```python
from build123d import *

# Parameters (mm, degrees)
BOSS_EXTRUDE1_DEPTH     = 1
SKETCH2_W               = 20
SKETCH2_H               = 30
BOSS_EXTRUDE2_DEPTH     = 1
MIRROR1_START           = 1
MIRROR1_DEPTH           = 1
MIRROR1_START_2         = 19
MIRROR1_2_DEPTH         = 1
FILLET1_R               = 1
CUT_EXTRUDE1_DEPTH      = 44.502679315
CUT_EXTRUDE1_DEPTH_BACK = 44.502679315
SKETCH3_R               = 2.5
CUT_EXTRUDE2_DEPTH      = 44.502679315
CUT_EXTRUDE2_DEPTH_BACK = 44.502679315
SKETCH4_W               = 27.584874686
SKETCH4_H               = 17.882608418


# Read off the part's stored shape, not the designer's step: Mirror1
with BuildPart() as part:
    # Sketch1 → Boss-Extrude1 (new body)
    with BuildSketch(Plane(origin=(0, 0, 0), x_dir=(0, 0, -1), z_dir=(1, 0, 0))):
        Polygon((0, 24.340975897), (30, 24.340975897), (0, -5.659024103), align=None)
    extrude(amount=BOSS_EXTRUDE1_DEPTH)

    # Sketch2 → Boss-Extrude2 (add)
    with BuildSketch(Plane(origin=(0, 24.340975897, 0), x_dir=(1, 0, 0), z_dir=(0, 1, 0))):
        with Locations((10, 15)):
            Rectangle(SKETCH2_W, SKETCH2_H)
    extrude(amount=-BOSS_EXTRUDE2_DEPTH)

    # Mirror1 outline → Mirror1 (add)
    with BuildSketch(Plane.YZ.offset(MIRROR1_START)):
        Polygon((-5.659024103, 0), (23.340975897, -29), (23.340975897, 0), align=None)
    extrude(amount=MIRROR1_DEPTH)

    # Mirror1 2 outline → Mirror1 2 (add)
    with BuildSketch(Plane.YZ.offset(MIRROR1_START_2)):
        Polygon((-5.659024103, 0), (23.340975897, -29), (23.340975897, 0), align=None)
    extrude(amount=MIRROR1_2_DEPTH)

    # Fillet1
    fillet1_edges = [part.edges().sort_by_distance(p)[0] for p in [
        (20, 24.340975897, -15),
        (19, 23.340975897, -14.5),
        (0, 24.340975897, -15),
        (2, 23.340975897, -14.5),
    ]]
    fillet(fillet1_edges, radius=FILLET1_R - 0.0001)  # a hair under: the kernel refuses the full size

    # Sketch3 → Cut-Extrude1 (cut, two sides: drawn at the far end of the back side and taken through both)
    with BuildSketch(Plane.ZY.offset(-CUT_EXTRUDE1_DEPTH_BACK)):
        with Locations((-5.377949805, 12.578820342)):
            Circle(SKETCH3_R)
    extrude(amount=CUT_EXTRUDE1_DEPTH + CUT_EXTRUDE1_DEPTH_BACK, mode=Mode.SUBTRACT)

    # Sketch4 → Cut-Extrude2 (cut, two sides: drawn at the far end of the back side and taken through both)
    with BuildSketch(Plane.ZY.offset(-CUT_EXTRUDE2_DEPTH_BACK)):
        with Locations((-7.379594799, -1.984577464)):
            Rectangle(SKETCH4_W, SKETCH4_H)
    extrude(amount=CUT_EXTRUDE2_DEPTH + CUT_EXTRUDE2_DEPTH_BACK, mode=Mode.SUBTRACT)


solid = part.part
```
Check sheet for the modelled part. Datum: model origin and axes. Units: mm. A direction names the side the tool comes from. Round coordinates to 2 decimals unless told otherwise and drop trailing zeros. Order: outer loops, then holes, each group sorted by start corner. A loop starts at its lowest first (then second) coordinate and runs counter-clockwise, first axis right, second up. Notation, with made-up numbers: M 8.5,70.5 L 38.5,70.5 A3 cw 38.5,75.5 Z; hole C -10.75,-35 d5. An arc over 180 degrees is marked long. Answer in a Markdown table with one row per item.
(1) Section check C-C on y = 14.5. Record the boundary of the cut face in (x, z).
Findings:
| item | result |
|---|---|
| outline | M 0,-20.16 L 2,-20.16 L 2,-6.98 L 0,-6.98 Z; M 0,-3.78 L 2,-3.78 L 2,0 L 0,0 Z; M 19,-20.16 L 20,-20.16 L 20,-6.98 L 19,-6.98 Z; M 19,-3.78 L 20,-3.78 L 20,0 L 19,0 Z |
(2) Material ranges on line 1 along X through (y, z) = (20.75, -25); line 2 along Y through (x, z) = (17, -3.5); line 3 along Z through (x, y) = (1, 12), recorded low to high. Write a range as from..to.
Findings:
| item | result |
|---|---|
| line 1 | x = 0..2, 19..20 |
| line 2 | y = 23.34..24.34 |
| line 3 | z = -17.66..-7.81, -2.95..0 |
(3) Section check A-A on z = -9. Record the boundary of the cut face in (x, y), plus the area to 3 significant figures.
Findings:
| item | result |
|---|---|
| outline | M 0,6.96 L 2,6.96 L 2,22.34 A1 cw 3,23.34 L 18,23.34 A1 cw 19,22.34 L 19,6.96 L 20,6.96 L 20,23.34 A1 ccw 19,24.34 L 1,24.34 A1 ccw 0,23.34 Z |
| area | 69.2 mm^2 |
(4) Gauge pin test, flat ends, axial feed: pin 1 (4 mm diameter, centred on x = 16, z = -13, fed in from -Y); pin 2 (4.5 mm diameter, centred on y = 12.58, z = -5.38, fed in from +X); pin 3 (4 mm diameter, centred on x = 3, z = -24, fed in from -Y). Record the tip position at first contact, or that the pin passes through.
Findings:
| item | result |
|---|---|
| pin 1 | stops at y = 23.34 |
| pin 2 | passes through |
| pin 3 | stops at y = 16.61 |
(5) Section check B-B on y = 17.5. Record the boundary of the cut face in (x, z), plus the area to 3 significant figures.
Findings:
| item | result |
|---|---|
| outline | M 0,-23.16 L 2,-23.16 L 2,0 L 0,0 Z; M 19,-23.16 L 20,-23.16 L 20,0 L 19,0 Z |
| area | 69.5 mm^2 |
(6) Draft check along X on faces 1 (the flat face through (1, 6.957, -6)), 2 (the cylindrical face through (19.715, 24.04, -15.21)), 3 (the cylindrical face through (18.715, 23.04, -14.297)). Enter one of: +X half, -X half, draft (parallel to the pull), parting line (faces both ways), or undercut.
Findings:
| item | result |
|---|---|
| face 1 | draft |
| face 2 | +X half |
| face 3 | undercut |
(7) Set-up check for faces 4 (the flat face through (19, 16, -11)), 5 (the flat face through (10, 24, -30)): record each of +Z, -Z, +X, -X, +Y, -Y from which the full face is reachable in a straight line by a thin tool's end or side.
Findings:
| item | result |
|---|---|
| face 4 | +Z, -Z, -Y |
| face 5 | -Z, +X, -X, +Y, -Y |
(8) Section check D-D on z = -4. Record the boundary of the cut face in (x, y), plus the area to 3 significant figures.
Findings:
| item | result |
|---|---|
| outline | M 0,6.96 L 2,6.96 L 2,10.49 L 0,10.49 Z; M 0,14.66 L 2,14.66 L 2,22.34 A1 cw 3,23.34 L 18,23.34 A1 cw 19,22.34 L 19,14.66 L 20,14.66 L 20,23.34 A1 ccw 19,24.34 L 1,24.34 A1 ccw 0,23.34 Z; M 19,6.96 L 20,6.96 L 20,10.49 L 19,10.49 Z |
| area | 56.6 mm^2 |
